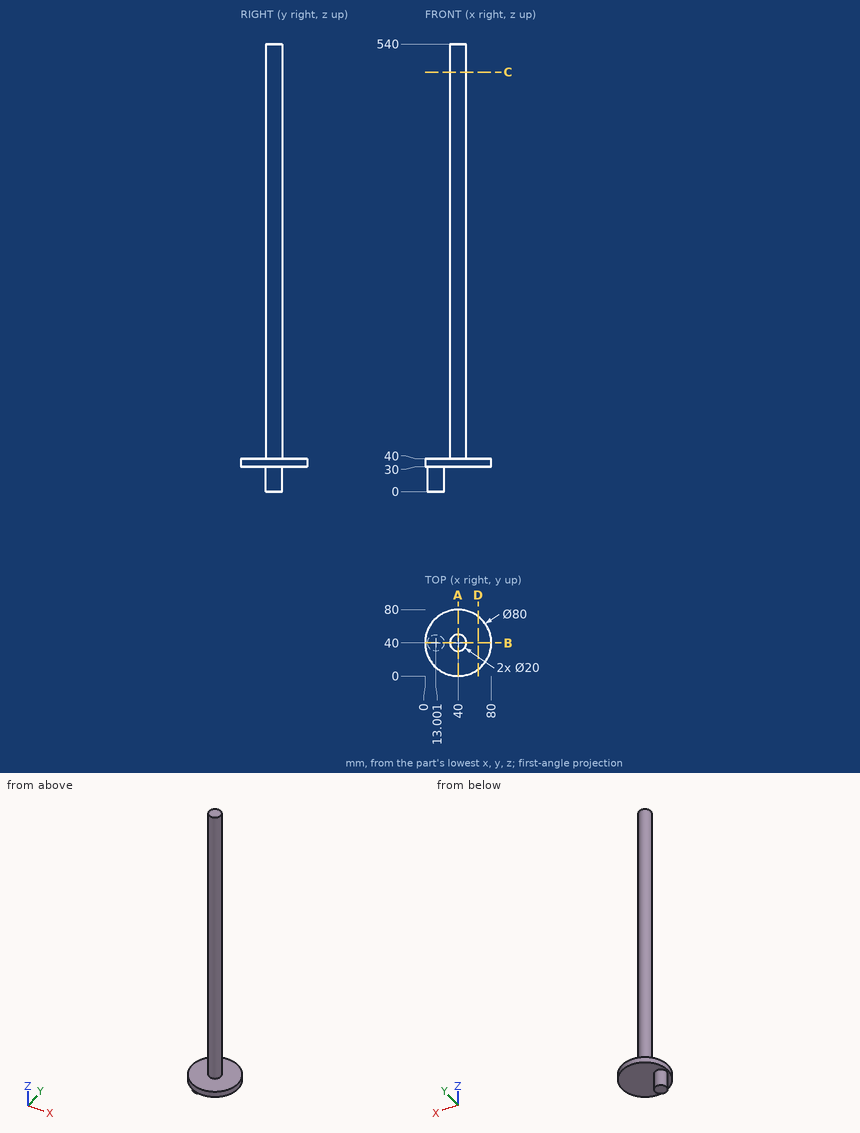
Verification items for this drawing (mm, ordinates from the low corner). Give positions to 0.01 mm unless a question says otherwise; leave off trailing zeros. Order: outer loops, then holes, each group sorted by start corner. A loop starts at its lowest first (then second) coordinate and runs counter-clockwise, first axis right, second up.
1) Cross-section at B-B (y = 40). Record the boundary of the cut face in (x, z), then the cut area to 3 significant figures.
Results are:
outline: (0, 30) - (3, 30) - (3, 0) - (23, 0) - (23, 30) - (80, 30) - (80, 40) - (50, 40) - (50, 540) - (30, 540) - (30, 40) - (0, 40) - close
area: 11,400 mm2
2) Gauge pin test, flat ends, axial feed: pin 1 (3 mm diameter, centred on x = 32, y = 55.5, fed in from -Z); pin 2 (10 mm diameter, centred on y = 51.5, z = 82.5, fed in from -X); pin 3 (10 mm diameter, centred on y = 41, z = 73.5, fed in from +X). Record the tip position at first contact, or that the pin passes through.
Results are:
pin 1: stops at z = 30
pin 2: stops at x = 32.4
pin 3: stops at x = 50
3) Cross-section at A-A (x = 40). Record the boundary of the cut face in (y, z).
Results are:
outline: (0, 30) - (80, 30) - (80, 40) - (50, 40) - (50, 540) - (30, 540) - (30, 40) - (0, 40) - close
4) Cross-section at D-D (x = 64). Record the boundary of the cut face in (y, z), then the cut area to 3 significant figures.
Results are:
outline: (8, 30) - (72, 30) - (72, 40) - (8, 40) - close
area: 640 mm2
5) Cross-section at C-C (z = 506). Record the boundary of the cut face in (x, y), then the cut area to 3 significant figures.
Results are:
outline: circle Ø20 at (40, 40)
area: 314 mm2
6) Material ranges on probe 1 along Z at (x, y) = (13.5, 60.5); probe 2 along Y at (x, z) = (41, 281.5); probe 3 along Z at (x, y) = (15.5, 45), recorded low to high.
Results are:
probe 1: z = 30 to 40
probe 2: y = 30.05 to 49.95
probe 3: z = 0 to 40
